The model under review builds one solid part; all positions refer to its coordinate system, in mm. Face numbers are marked on the shaded views. Round coordinates to 2 decimals unless told otherwise and drop trailing zeros. Order: outer loops, then holes, each group sorted by start corner. A loop starts at its lowest first (then second) coordinate and runs counter-clockwise, first axis right, second up. Notation, with made-up numbers: M -30,52 L 5,52 A32 cw 5,84 Z; hole C 49,10 d4. An arc over 180 degrees is marked long. Answer as a JSON object with one key per item and string values. Group by question number.
1) The part is to be moulded in two halves that separate along X. For the marked faces 1 and 2, say which applies: +X half, -X half, draft (parallel to the pull), parting line (faces both ways), or undercut.
2) To check wall thickness, follow line 1 (X direction, y = 1.6, z = 8); line 2 (Y direction, x = 1.15, z = -36.65) (3 decimals); line 3 (X direction, y = 2, z = 0). State the ranges of each line that lie inside material, in increasing order.
3) Insertion check: pin 1 Ø4 at (x, z) = (9.23, -8) entering from -Y; pin 2 Ø10 at (x, z) = (15, 18) entering from +Y. Each pin has a flat end and moves straight along its axis. Give the tip position at first contact, or say it passes through.
4) Consider section D-D, the plane z = 17. Write out the cut boundary in (x, y), then the cut area to 3 significant figures.
5) Consider section C-C, the plane y = 7.25. Write out the cut boundary in (x, z), then the cut area to 3 significant figures.
6) Consider section A-A, the plane z = -8. Write out the cut boundary in (x, y).
7) Consider section B-B, the plane x = 9.23. Write out the cut boundary in (y, z), then the cut area to 3 significant figures.
```python
from build123d import *

# Parameters (mm, degrees)
EXTRUDE_THIN1_DEPTH = 50
CUT_EXTRUDE2_REACH  = 58.796
SKETCH4_R           = 4
SKETCH3_R           = 5.1
SKETCH3_R_2         = 1.5
CUT_EXTRUDE1_DEPTH  = 3


with BuildPart() as part:
    # Sketch1 → Extrude-Thin1 (new, symmetric)
    with BuildSketch(Plane.XY):
        Polygon((19.05, 0), (0, 0), (0, 19.05), (3, 19.05), (3, 3), (19.05, 3), align=None)
    extrude(amount=EXTRUDE_THIN1_DEPTH, both=True)

    # Sketch4 → Cut-Extrude2 (cut, up to next)
    with BuildSketch(Plane.ZY, mode=Mode.PRIVATE) as cut_extrude2_sk1:
        with Locations((-36.65, 9.525)):
            Circle(SKETCH4_R)
    cut_extrude2_tool1 = extrude(cut_extrude2_sk1.sketch, amount=-CUT_EXTRUDE2_REACH, mode=Mode.PRIVATE) & part.part
    # Sketch4 → Cut-Extrude2 (cut, up to next)
    with BuildSketch(Plane.ZY, mode=Mode.PRIVATE) as cut_extrude2_sk2:
        with Locations((36.65, 9.525)):
            Circle(SKETCH4_R)
    cut_extrude2_tool2 = extrude(cut_extrude2_sk2.sketch, amount=-CUT_EXTRUDE2_REACH, mode=Mode.PRIVATE) & part.part
    add(cut_extrude2_tool1.solids().sort_by_distance((0, 9.525, -36.65))[0], mode=Mode.SUBTRACT)
    add(cut_extrude2_tool2.solids().sort_by_distance((0, 9.525, 36.65))[0], mode=Mode.SUBTRACT)

    # Sketch3 → Cut-Extrude1 (cut)
    with BuildSketch(Plane.XZ):
        with Locations(Location((9.23, 0, 0), (0, 0, 270))):
            Circle(SKETCH3_R)
        with Locations(Location((9.23, -8, 0), (0, 0, 270))):
            Circle(SKETCH3_R_2)
        with Locations(Location((9.23, 8, 0), (0, 0, 270))):
            Circle(SKETCH3_R_2)
    extrude(amount=-CUT_EXTRUDE1_DEPTH, mode=Mode.SUBTRACT)


solid = part.part
```
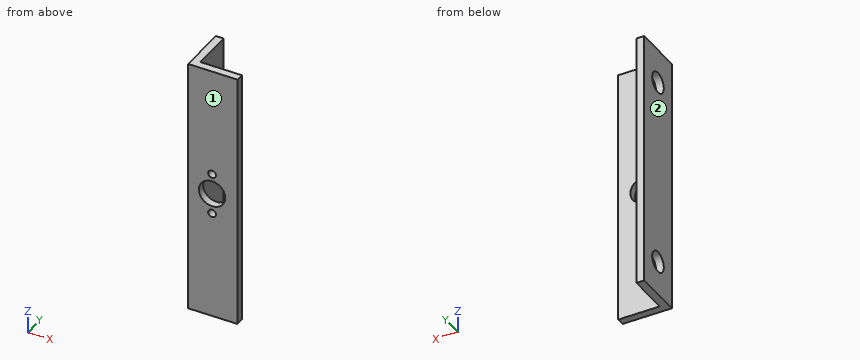
Results list:
{
 "1": {"face 1": "draft", "face 2": "-X half"},
 "2": {"line 1": "0 to 7.73, 10.73 to 19.05", "line 2": "0 to 5.525, 13.525 to 19.05", "line 3": "0 to 4.13, 14.33 to 19.05"},
 "3": {"pin 1": "y = 0", "pin 2": "y = 3"},
 "4": {"outline": "M 0,0 L 19.05,0 L 19.05,3 L 3,3 L 3,19.05 L 0,19.05 Z", "area": "105 mm^2"},
 "5": {"outline": "M 0,-50 L 3,-50 L 3,-39.94 L 0,-39.94 Z; M 0,-33.36 L 3,-33.36 L 3,33.36 L 0,33.36 Z; M 0,39.94 L 3,39.94 L 3,50 L 0,50 Z", "area": "261 mm^2"},
 "6": {"outline": "M 0,0 L 7.73,0 L 7.73,3 L 3,3 L 3,19.05 L 0,19.05 Z; M 10.73,0 L 19.05,0 L 19.05,3 L 10.73,3 Z"},
 "7": {"outline": "M 0,-50 L 3,-50 L 3,-9.5 L 0,-9.5 Z; M 0,-6.5 L 3,-6.5 L 3,-5.1 L 0,-5.1 Z; M 0,5.1 L 3,5.1 L 3,6.5 L 0,6.5 Z; M 0,9.5 L 3,9.5 L 3,50 L 0,50 Z", "area": "251 mm^2"}
}
